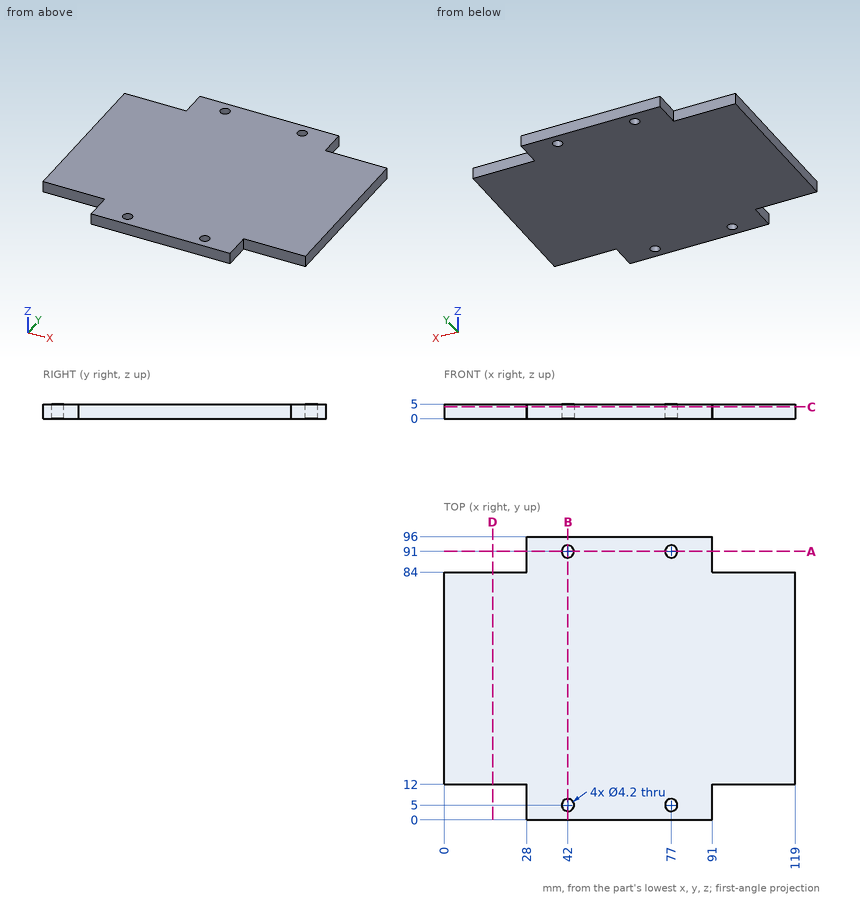
Here's the drawing with two shaded views (mm, measured from the low corner). I have some questions. Round coordinates to 2 decimals unless told otherwise and drop trailing zeros. Order: outer loops, then holes, each group sorted by start corner. A loop starts at its lowest first (then second) coordinate and runs counter-clockwise, first axis right, second up. Notation, with made-up numbers: M 81.5,-36 L 89.5,-36 A31 cw 89.5,-5 Z; hole C 36,65 d2. An arc over 180 degrees is marked long. Use CSV: the item, a comma, the result in double quotes.
1) I need wall thicknesses on line 1 along Y through (x, z) = (77, 2.5); line 2 along Y through (x, z) = (10.5, 1.95); line 3 along X through (y, z) = (6, 4.25). Which ranges of each line are inside material? Lowest first, please. Write a range as [from, to].
Taken from the geometry:
line 1,"[0, 2.9], [7.1, 88.9], [93.1, 96]"
line 2,"[12, 84]"
line 3,"[28, 40.15], [43.85, 75.15], [78.85, 91]"
2) I want a section at B-B (x = 42). List the corners of the cut face in (y, z) for me.
Taken from the geometry:
outline,"M 0,0 L 2.9,0 L 2.9,5 L 0,5 Z; M 7.1,0 L 88.9,0 L 88.9,5 L 7.1,5 Z; M 93.1,0 L 96,0 L 96,5 L 93.1,5 Z"
3) I'm going to push flat-ended pins straight in: P1, Ø4, axis at x = 42, y = 5, coming from the -Z side; P2, Ø1.5, axis at x = 16.5, z = 3.5, coming from the -Y side; P3, Ø1.5, axis at y = 89.5, z = 3, coming from the -X side. Where does each tip first touch, or does it pass through?
Taken from the geometry:
P1,"through"
P2,"y = 12"
P3,"x = 28"
4) I want a section at A-A (y = 91). List the corners of the cut face in (x, z) for me.
Taken from the geometry:
outline,"M 28,0 L 39.9,0 L 39.9,5 L 28,5 Z; M 44.1,0 L 74.9,0 L 74.9,5 L 44.1,5 Z; M 79.1,0 L 91,0 L 91,5 L 79.1,5 Z"
5) I want a section at D-D (x = 16.5). List the corners of the cut face in (y, z) for me.
Taken from the geometry:
outline,"M 12,0 L 84,0 L 84,5 L 12,5 Z"
6) I want a section at C-C (z = 4.05). List the corners of the cut face in (x, y) for me.
Taken from the geometry:
outline,"M 0,12 L 28,12 L 28,0 L 91,0 L 91,12 L 119,12 L 119,84 L 91,84 L 91,96 L 28,96 L 28,84 L 0,84 Z; hole C 42,5 d4.2; hole C 42,91 d4.2; hole C 77,5 d4.2; hole C 77,91 d4.2"
